```python
from build123d import *

# Parameters (mm, degrees)
SKETCH1_W               = 80
SKETCH1_H               = 90
BOSS_EXTRUDE1_DEPTH     = 6
SKETCH4_W               = 80
SKETCH4_H               = 90
SKETCH4_W_2             = 73
SKETCH4_H_2             = 83
BOSS_EXTRUDE2_DEPTH     = 34
SKETCH6_R               = 4.05
CUT_EXTRUDE1_DEPTH      = 40
SKETCH7_R               = 7
CUT_EXTRUDE2_DEPTH      = 2.8
BOSS_EXTRUDE3_DEPTH     = 7
SKETCH11_R              = 2.85
BOSS_EXTRUDE4_DEPTH     = 2
CUT_EXTRUDE3_DEPTH      = 9
CUT_EXTRUDE3_DEPTH_BACK = 6
SKETCH5_R               = 1.5
CUT_EXTRUDE4_DEPTH      = 6
CUT_EXTRUDE4_DEPTH_BACK = 70.144775652
SKETCH12_W              = 18
SKETCH12_H              = 15
CUT_EXTRUDE6_DEPTH      = 3.5
SKETCH17_R              = 8
CUT_EXTRUDE8_DEPTH      = 2
CUT_EXTRUDE9_DEPTH      = 1.5
CUT_EXTRUDE14_DEPTH     = 10
SKETCH30_R              = 2
CUT_EXTRUDE15_DEPTH     = 10
BOSS_EXTRUDE6_DEPTH     = 4
CUT_EXTRUDE12_DEPTH     = 4
SKETCH26_R              = 4
CUT_EXTRUDE13_DEPTH     = 4


with BuildPart() as part:
    # Sketch1 → Boss-Extrude1 (new body)
    with BuildSketch(Plane(origin=(0, 0, 0), x_dir=(1, 0, 0), z_dir=(0, 1, 0))):
        Rectangle(SKETCH1_W, SKETCH1_H)
    extrude(amount=BOSS_EXTRUDE1_DEPTH)

    # Sketch4 → Boss-Extrude2 (add)
    with BuildSketch(Plane(origin=(0, 6, 0), x_dir=(1, 0, 0), z_dir=(0, 1, 0))):
        Rectangle(SKETCH4_W, SKETCH4_H)
        Rectangle(SKETCH4_W_2, SKETCH4_H_2, mode=Mode.SUBTRACT)
    extrude(amount=BOSS_EXTRUDE2_DEPTH)

    # Sketch6 → Cut-Extrude1 (cut)
    with BuildSketch(Plane(origin=(0, 6, 0), x_dir=(1, 0, 0), z_dir=(0, 1, 0))):
        with Locations(Location((-20, 17, 0), (0, 0, 270))):
            Circle(SKETCH6_R)
        with Locations(Location((-20, -25, 0), (0, 0, 270))):
            Circle(SKETCH6_R)
    extrude(amount=-CUT_EXTRUDE1_DEPTH, mode=Mode.SUBTRACT)

    # Sketch7 → Cut-Extrude2 (cut)
    with BuildSketch(Plane(origin=(0, 6, 0), x_dir=(1, 0, 0), z_dir=(0, 1, 0))):
        with Locations(Location((-20, 17, 0), (0, 0, 270))):
            Circle(SKETCH7_R)
        with Locations(Location((-20, -25, 0), (0, 0, 270))):
            Circle(SKETCH7_R)
    extrude(amount=-CUT_EXTRUDE2_DEPTH, mode=Mode.SUBTRACT)

    # Sketch10 → Boss-Extrude3 (add)
    with BuildSketch(Plane(origin=(0, 6, 0), x_dir=(1, 0, 0), z_dir=(0, 1, 0))):
        Polygon((-32.5, 43.100297611), (-37.35, 40.300148806), (-37.35, 34.699851194), (-32.5, 31.899702389), (-27.65, 34.699851194), (-27.65, 40.300148806), align=None)
        Polygon((-27.65, 9.300148806), (-32.5, 12.100297611), (-37.35, 9.300148806), (-37.35, 3.699851194), (-32.5, 0.899702389), (-27.65, 3.699851194), align=None)
    extrude(amount=BOSS_EXTRUDE3_DEPTH)

    # Sketch11 → Boss-Extrude4 (add)
    with BuildSketch(Plane(origin=(0, 13, 0), x_dir=(1, 0, 0), z_dir=(0, 1, 0))):
        with Locations(Location((-32.5, 37.5, 0), (0, 0, 270))):
            Circle(SKETCH11_R)
        with Locations(Location((-32.5, 6.5, 0), (0, 0, 270))):
            Circle(SKETCH11_R)
    extrude(amount=BOSS_EXTRUDE4_DEPTH)

    # Sketch5 → Cut-Extrude3 (cut, two sides: drawn at the far end of the back side and taken through both)
    with BuildSketch(Plane(origin=(0, 6, 0), x_dir=(1, 0, 0), z_dir=(0, 1, 0)).offset(-CUT_EXTRUDE3_DEPTH_BACK)):
        with Locations(Location((-32.5, 37.5, 0), (0, 0, 270))):
            Circle(SKETCH5_R)
        with Locations(Location((-32.5, 6.5, 0), (0, 0, 270))):
            Circle(SKETCH5_R)
    extrude(amount=CUT_EXTRUDE3_DEPTH + CUT_EXTRUDE3_DEPTH_BACK, mode=Mode.SUBTRACT)

    # Sketch8 → Cut-Extrude4 (cut, two sides: drawn at the far end of the back side and taken through both)
    with BuildSketch(Plane(origin=(0, 6, 0), x_dir=(1, 0, 0), z_dir=(0, 1, 0)).offset(-CUT_EXTRUDE4_DEPTH_BACK)):
        Polygon((-29.65, 39.145448267), (-32.5, 40.790896534), (-35.35, 39.145448267), (-35.35, 35.854551733), (-32.5, 34.209103466), (-29.65, 35.854551733), align=None)
        Polygon((-29.65, 8.145448267), (-32.5, 9.790896534), (-35.35, 8.145448267), (-35.35, 4.854551733), (-32.5, 3.209103466), (-29.65, 4.854551733), align=None)
    extrude(amount=CUT_EXTRUDE4_DEPTH + CUT_EXTRUDE4_DEPTH_BACK, mode=Mode.SUBTRACT)

    # Sketch12 → Cut-Extrude6 (cut)
    with BuildSketch(Plane(origin=(-36.5, 0, 0), x_dir=(0, 0, -1), z_dir=(1, 0, 0))):
        with Locations((22, 24)):
            Rectangle(SKETCH12_W, SKETCH12_H)
    extrude(amount=-CUT_EXTRUDE6_DEPTH, mode=Mode.SUBTRACT)

    # Sketch17 → Cut-Extrude8 (cut)
    with BuildSketch(Plane.ZY.offset(40)):
        with Locations((29.75, 20)):
            Circle(SKETCH17_R)
    extrude(amount=-CUT_EXTRUDE8_DEPTH, mode=Mode.SUBTRACT)

    # Sketch15 → Cut-Extrude9 (cut)
    with BuildSketch(Plane(origin=(-36.5, 0, 0), x_dir=(0, 0, -1), z_dir=(1, 0, 0))):
        Polygon((-29.75, 32.990381057), (-41, 26.495190528), (-41, 13.504809472), (-29.75, 7.009618943), (-18.5, 13.504809472), (-18.5, 26.495190528), align=None)
    extrude(amount=-CUT_EXTRUDE9_DEPTH, mode=Mode.SUBTRACT)

    # Sketch29 → Cut-Extrude14 (cut)
    with BuildSketch(Plane(origin=(0, 6, 0), x_dir=(1, 0, 0), z_dir=(0, 1, 0))):
        with BuildLine():
            Line((8, 18.9), (8, 8.1))
            ThreePointArc((8, 8.1), (4, 4.1), (0, 8.1))
            Line((0, 8.1), (0, 18.9))
            ThreePointArc((0, 18.9), (4, 22.9), (8, 18.9))
        make_face()
    extrude(amount=-CUT_EXTRUDE14_DEPTH, mode=Mode.SUBTRACT)

    # Sketch30 → Cut-Extrude15 (cut)
    with BuildSketch(Plane(origin=(40, 0, 0), x_dir=(0, 0, -1), z_dir=(1, 0, 0))):
        with Locations((-33.5, 20)):
            Circle(SKETCH30_R)
        with Locations((-16.5, 20)):
            Circle(SKETCH30_R)
        with BuildLine():
            Line((-28.5, 22), (-21.5, 22))
            ThreePointArc((-21.5, 22), (-19.5, 20), (-21.5, 18))
            Line((-21.5, 18), (-28.5, 18))
            ThreePointArc((-28.5, 18), (-30.5, 20), (-28.5, 22))
        make_face()
    extrude(amount=-CUT_EXTRUDE15_DEPTH, mode=Mode.SUBTRACT)

    # Sketch23 → Boss-Extrude6 (add)
    with BuildSketch(Plane(origin=(0, 40, 0), x_dir=(1, 0, 0), z_dir=(0, 1, 0))):
        Polygon((-10, -45), (-40, -5), (-40, -45), align=None)
        Polygon((40, -45), (10, -45), (40, -5), align=None)
        Polygon((-40, 45), (-40, 15), (-10, 45), align=None)
        Polygon((10, 45), (40, 45), (40, 15), align=None)
    extrude(amount=-BOSS_EXTRUDE6_DEPTH)

    # Sketch27 → Cut-Extrude12 (cut)
    with BuildSketch(Plane(origin=(0, 40, 0), x_dir=(1, 0, 0), z_dir=(0, 1, 0))):
        with BuildLine():
            Line((-30.5, 37.5), (-30.5, 30.5))
            ThreePointArc((-30.5, 30.5), (-32.5, 28.5), (-34.5, 30.5))
            Line((-34.5, 30.5), (-34.5, 37.5))
            ThreePointArc((-34.5, 37.5), (-32.5, 39.5), (-30.5, 37.5))
        make_face()
        with BuildLine():
            Line((34.5, 37.5), (34.5, 30.5))
            ThreePointArc((34.5, 30.5), (32.5, 28.5), (30.5, 30.5))
            Line((30.5, 30.5), (30.5, 37.5))
            ThreePointArc((30.5, 37.5), (32.5, 39.5), (34.5, 37.5))
        make_face()
        with BuildLine():
            Line((34.5, -29), (34.5, -36))
            ThreePointArc((34.5, -36), (32.5, -38), (30.5, -36))
            Line((30.5, -36), (30.5, -29))
            ThreePointArc((30.5, -29), (32.5, -27), (34.5, -29))
        make_face()
        with BuildLine():
            Line((-30.5, -29), (-30.5, -36))
            ThreePointArc((-30.5, -36), (-32.5, -38), (-34.5, -36))
            Line((-34.5, -36), (-34.5, -29))
            ThreePointArc((-34.5, -29), (-32.5, -27), (-30.5, -29))
        make_face()
    extrude(amount=-CUT_EXTRUDE12_DEPTH, mode=Mode.SUBTRACT)

    # Sketch26 → Cut-Extrude13 (cut)
    with BuildSketch(Plane(origin=(0, 40, 0), x_dir=(1, 0, 0), z_dir=(0, 1, 0))):
        with Locations((-32.5, 37.5)):
            Circle(SKETCH26_R)
        with Locations((32.5, 37.5)):
            Circle(SKETCH26_R)
        with Locations((32.5, -29)):
            Circle(SKETCH26_R)
        with Locations((-32.5, -29)):
            Circle(SKETCH26_R)
    extrude(amount=-CUT_EXTRUDE13_DEPTH, mode=Mode.SUBTRACT)


solid = part.part
```
Could you check a few things on this model? Use its own coordinates, in mm. A direction names the side the tool comes from. Give positions to 0.01 mm unless a question says otherwise; leave off trailing zeros. Write each loop counter-clockwise with the first axis right and the second up, starting at its lowest first coordinate (ties: lowest second). Pieces come first, ordered by that corner, then holes. Notation, with made-up numbers: (42, 37) - (77, 37) arc R8 cw to (77, 46) - close; hole circle Ø1 at (73.5, 27.25). An arc over 180 degrees is marked (long way). One line per item, written item: value. Start each with the question number.
Item 1: Which directions (+Z, -Z, +X, -X, +Y, -Y) give clear straight access to the entire face, cutting with the end or side of a thin tool? Please do faces 3 (the face through (-23, 3.2, 28)), 4 (the face through (-38, 24, -13)), 5 (the face through (8, 3, -14)), 6 (the face through (24.4, 38, 25.8)), 7 (the face through (-33.2, 12, -8)).
Item 2: Please list where these lines run through material, in increasing order: line 1 (X direction, y = 13.3, z = -6.5); line 2 (Z direction, x = -32.5, y = 12.9); line 3 (Y direction, x = 33.5, z = -26). Write a range as from..to.
Item 3: Imagine slicing it at B-B, the plane y = 23.5. List the corners of the cut face in (x, z) for me, and give its area (3 significant figures).
Item 4: Imagine slicing it at A-A, the plane z = -17. List the corners of the cut face in (x, y) for me, and give its area (3 significant figures).
Item 5: If we mould it in two halves opening along Z, with no side actions, what happens to faces 1 (the face through (-40, 20, 1)), 2 (the face through (-37.24, 29.7, 24.05))? For each: +Z half, -Z half, draft (parallel to the pull), parting line (faces both ways), or undercut.
Item 6: Imagine slicing it at D-D, the plane z = 33.5. Give the number of separate pieces and of enclosed holes in the cut face, and give its area (3 significant figures).
Item 7: Imagine slicing it at C-C, the plane x = -10. List the corners of the cut face in (y, z) for me, and give its area (3 significant figures).
Item 8: I'm going to push flat-ended pins straight in: pin 1 (3.5 mm diameter, centred on x = -32.5, z = -6.5, fed in from +Y); pin 2 (6 mm diameter, centred on x = -18.5, z = 5.5, fed in from +Y). Where does each tip first touch, or does it pass through?
Geometry says:
1. face 3: none
1. face 4: -X
1. face 5: +Y, -Y
1. face 6: +Y
1. face 7: -Y
2. line 1: -40..-36.5, -35.35..-34, -31..-29.65, 36.5..40
2. line 2: -45..-39, -36..-31.9, -12.1..-8, -5..-0.9, 41.5..45
2. line 3: 0..6, 36..40
3. outline: (-40, -45) - (40, -45) - (40, 45) - (-40, 45) - (-40, 36.94) - (-38, 36.94) - (-38, 41) - (-36.5, 41) - (-36.5, 41.5) - (36.5, 41.5) - (36.5, -41.5) - (-36.5, -41.5) - (-36.5, -31) - (-40, -31) - close; (-40, -13) - (-36.5, -13) - (-36.5, 18.5) - (-38, 18.5) - (-38, 22.56) - (-40, 22.56) - close
3. area: 1,020 mm^2
4. outline: (-40, 0) - (-24.05, 0) - (-24.05, 3.2) - (-27, 3.2) - (-27, 6) - (-36.5, 6) - (-36.5, 16.5) - (-40, 16.5) - close; (-40, 31.5) - (-36.5, 31.5) - (-36.5, 40) - (-40, 40) - close; (-15.95, 0) - (0, 0) - (0, 6) - (-13, 6) - (-13, 3.2) - (-15.95, 3.2) - close; (8, 0) - (40, 0) - (40, 40) - (36.5, 40) - (36.5, 6) - (8, 6) - close
4. area: 552 mm^2
5. face 1: draft
5. face 2: undercut
6. separate pieces: 5
6. enclosed holes: 0
6. area: 754 mm^2
7. outline: (0, -45) - (40, -45) - (40, -41.5) - (6, -41.5) - (6, 41.5) - (40, 41.5) - (40, 45) - (0, 45) - close
7. area: 778 mm^2
8. pin 1: y = 15
8. pin 2: y = 6
